The listing builds one solid part. Answer for the finished solid, in the listing's coordinates (mm). Face numbers are marked on the shaded views. A direction names the side the tool comes from. Round coordinates to 2 decimals unless told otherwise and drop trailing zeros. Order: outer loops, then holes, each group sorted by start corner. A loop starts at its lowest first (then second) coordinate and runs counter-clockwise, first axis right, second up. Notation, with made-up numbers: (-15.75, -30.5) -> (10.25, -30.5) arc R15 ccw to (10.25, -9.5) -> close; hole circle Ø8 at (77.25, 33.25). An arc over 180 degrees is marked (long way). Return JSON: item names as keys, results as strings. Group by question number.
(1) The part is cut by section B-B (z = 9). Determine the outline of the cut face in (x, y), plus the area to 3 significant figures.
(2) Consider line 1 (Y direction, x = 20, z = 8.75); line 2 (Y direction, x = 34, z = 3.75); line 3 (Z direction, x = 18, y = 5.25). Determine where each line is inside the solid, lowest interval first. Write a range as [from, to].
(3) The part is cut by section D-D (z = 6.75). Determine the outline of the cut face in (x, y), plus the area to 3 significant figures.
(4) Determine the mould class of the marked faces 1, 2, 3 and 4 for opening direction Y: +Y half, -Y half, draft (parallel to the pull), parting line (faces both ways), or undercut.
(5) The part is cut by section C-C (y = 8.25). Determine the outline of the cut face in (x, z), plus the area to 3 significant figures.
(6) Each of these flat-tipped pins is pushed along its axis until it touches: pin 1 (5 mm diameter, centred on y = 12, z = 1.5, fed in from -X); pin 2 (1.2 mm diameter, centred on y = 21.5, z = 9.5, fed in from -X); pin 3 (7 mm diameter, centred on x = 35, y = 14.5, fed in from -Z); pin 4 (12 mm diameter, centred on x = 12, y = 4.5, fed in from -Z). Where does it stop, or does it pass through?
(7) Which of the six approach directions +Z, -Z, +X, -X, +Y, -Y give full straight-line access (tool end or side, diameter ignored) to the marked faces 5 and 6?
(8) The part is cut by section A-A (x = 36). Determine the outline of the cut face in (y, z).
from build123d import *

# Parameters (mm, degrees)
BOX_W           = 49.18
BOX_H           = 23.8
BOX_DEPTH       = 5
SKETCH_W        = 43.2
SKETCH_H        = 17.8
POCKET_DEPTH    = 2
SKETCH001_W     = 3
SKETCH001_H     = 9
POCKET002_DEPTH = 2
BOX001_W        = 51
BOX001_H        = 28
BOX001_DEPTH    = 10
SKETCH002_W     = 23.8
SKETCH002_H     = 5.5
POCKET003_DEPTH = 49.18
SKETCH003_W     = 47
SKETCH003_H     = 4
POCKET004_DEPTH = 5


with BuildPart() as pocket002:
    # Box → Box (new body)
    with BuildSketch(Plane.XY):
        with Locations((24.59, 11.9)):
            Rectangle(BOX_W, BOX_H)
    extrude(amount=BOX_DEPTH)

    # Sketch → Pocket (cut)
    with BuildSketch(Plane.XY.offset(5)):
        with Locations((24.6, 11.9)):
            Rectangle(SKETCH_W, SKETCH_H)
    extrude(amount=-POCKET_DEPTH, mode=Mode.SUBTRACT)

    # Sketch001 → Pocket002 (cut)
    with BuildSketch(Plane.XY.offset(5)):
        with Locations((1.5, 11.9)):
            Rectangle(SKETCH001_W, SKETCH001_H)
    extrude(amount=-POCKET002_DEPTH, mode=Mode.SUBTRACT)


with BuildPart() as pocket004:
    # Box001 → Box001 (new body)
    with BuildSketch(Plane(origin=(0, -2, 0), x_dir=(1, 0, 0), z_dir=(0, 0, 1))):
        with Locations((25.5, 14)):
            Rectangle(BOX001_W, BOX001_H)
    extrude(amount=BOX001_DEPTH)

    # Cut: cut Pocket002
    add(pocket002.part, mode=Mode.SUBTRACT)

    # Sketch002 → Pocket003 (cut)
    with BuildSketch(Plane(origin=(0, 0, 0), x_dir=(0, -1, 0), z_dir=(-1, 0, 0))):
        with Locations((-11.9, 5.75)):
            Rectangle(SKETCH002_W, SKETCH002_H)
    extrude(amount=-POCKET003_DEPTH, mode=Mode.SUBTRACT)

    # Sketch003 → Pocket004 (cut)
    with BuildSketch(Plane.XY.offset(10)):
        with Locations((23.5, 20.8)):
            Rectangle(SKETCH003_W, SKETCH003_H)
        with Locations((23.5, 3.2)):
            Rectangle(SKETCH003_W, SKETCH003_H)
    extrude(amount=-POCKET004_DEPTH, mode=Mode.SUBTRACT)


solid = pocket004.part
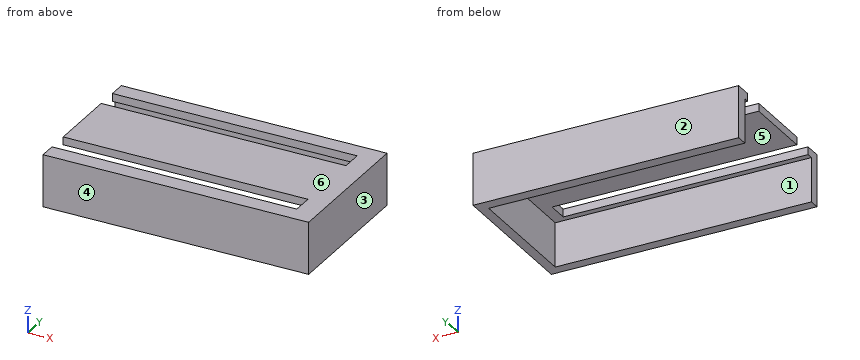
Answer below:
{
 "1": {"outline": "(0, -2) -> (51, -2) -> (51, 26) -> (0, 26) -> (0, 22.8) -> (47, 22.8) -> (47, 18.8) -> (0, 18.8) -> (0, 5.2) -> (47, 5.2) -> (47, 1.2) -> (0, 1.2) -> close", "area": "1,050 mm²"},
 "2": {"line 1": "y = [-2, 1.2], [5.2, 18.8], [22.8, 26]", "line 2": "y = [-2, 0], [23.8, 26]", "line 3": "z = [8.5, 10]"},
 "3": {"outline": "(0, -2) -> (51, -2) -> (51, 26) -> (0, 26) -> (0, 23.8) -> (49.18, 23.8) -> (49.18, 0) -> (0, 0) -> close", "area": "258 mm²"},
 "4": {"face 1": "undercut", "face 2": "+Y half", "face 3": "draft", "face 4": "-Y half"},
 "5": {"outline": "(0, 8.5) -> (49.18, 8.5) -> (49.18, 0) -> (51, 0) -> (51, 10) -> (0, 10) -> close", "area": "92.0 mm²"},
 "6": {"pin 1": "stops at x = 49.18", "pin 2": "stops at x = 47", "pin 3": "stops at z = 8.5", "pin 4": "stops at z = 0"},
 "7": {"face 5": "-Z, -X", "face 6": "+Z, +X, -X, +Y, -Y"},
 "8": {"outline": "(-2, 0) -> (0, 0) -> (0, 8.5) -> (1.2, 8.5) -> (1.2, 10) -> (-2, 10) -> close; (5.2, 8.5) -> (18.8, 8.5) -> (18.8, 10) -> (5.2, 10) -> close; (22.8, 8.5) -> (23.8, 8.5) -> (23.8, 0) -> (26, 0) -> (26, 10) -> (22.8, 10) -> close"}
}
